The listing builds one solid part. Answer for the finished solid, in the listing's coordinates (mm). A direction names the side the tool comes from. Round coordinates to 2 decimals unless told otherwise and drop trailing zeros. Write each loop counter-clockwise with the first axis right and the second up, starting at its lowest first coordinate (ties: lowest second). Pieces come first, ordered by that corner, then holes. Notation, with made-up numbers: M 39.25,-8.75 L 86.25,-8.75 A28 ccw 86.25,23.25 Z; hole C 31,0 d9. An arc over 180 degrees is marked long. One line per item, written item: value. Start each with the question number.
(1) Section B-B (x = 124.5) is taken. Determine the outline of the cut face in (y, z).
(2) Given P1, Ø10, axis at y = 3.5, z = -20, coming from the -X side; P2, Ø5, axis at y = 17, z = -32, coming from the -X side; P3, Ø3, axis at x = 81, y = 16, coming from the -Z side, each flat-ended and moving along its own axis, determine where each tip first touches the part or whether it passes through.
(3) Section D-D (z = -42) is taken. Determine the outline of the cut face in (x, y) (3 decimals), plus the area to 3 significant figures.
(4) Section C-C (y = 15.25) is taken. Determine the outline of the cut face in (x, z).
(5) Consider probe 1 along Y at (x, z) = (46.5, -7); probe 2 along X at (y, z) = (15, -19); probe 3 along Z at (x, y) = (181.5, 18.25). Determine where each line is inside the solid, lowest interval first.
(6) Section A-A (z = -10) is taken. Determine the outline of the cut face in (x, y) (3 decimals).
(7) For faces 1 (the flat face through (32.766, 16, -35)), 2 (the flat face through (126, 16, -52.07)), 3 (the flat face through (128, 16, -18.288)), determine the directions among +Z, -Z, +X, -X, +Y, -Y from which every point of the face is accessible in a straight line to the end or side of a thin tool.
```python
from build123d import *

# Parameters (mm, degrees)
SKETCH1_W           = 254
SKETCH1_H           = 58.42
BOSS_EXTRUDE1_DEPTH = 19.05
CUT_EXTRUDE1_DEPTH  = 6.35
FILLET1_R           = 9.525


with BuildPart() as part:
    # Sketch1 → Boss-Extrude1 (new body)
    with BuildSketch(Plane(origin=(0, 0, 0), x_dir=(1, 0, 0), z_dir=(0, 1, 0))):
        with Locations((127, 29.21)):
            Rectangle(SKETCH1_W, SKETCH1_H)
    extrude(amount=BOSS_EXTRUDE1_DEPTH)

    # Sketch2 → Cut-Extrude1 (cut)
    with BuildSketch(Plane(origin=(0, 19.05, 0), x_dir=(1, 0, 0), z_dir=(0, 1, 0))):
        Polygon((221.234, 52.07), (221.234, 18.288), (127, 18.288), (127, 0), (254, 0), (254, 58.42), (127, 58.42), (127, 52.07), align=None)
        Polygon((127, 0), (127, 18.288), (32.766, 18.288), (32.766, 52.07), (127, 52.07), (127, 58.42), (0, 58.42), (0, 0), align=None)
    extrude(amount=-CUT_EXTRUDE1_DEPTH, mode=Mode.SUBTRACT)

    # Fillet1
    fillet1_edges = [part.edges().sort_by_distance(p)[0] for p in [
        (254, 0, -29.21),
        (0, 0, -29.21),
    ]]
    fillet(fillet1_edges, radius=FILLET1_R)


solid = part.part
```
Recorded:
1. outline: M 0,-58.42 L 12.7,-58.42 L 12.7,-52.07 L 19.05,-52.07 L 19.05,-18.29 L 12.7,-18.29 L 12.7,0 L 0,0 Z
2. P1: stops at x = 0.06
2. P2: stops at x = 32.77
2. P3: stops at z = -52.07
3. outline: M 0,9.525 A9.525 ccw 9.525,0 L 244.475,0 A9.525 ccw 254,9.525 L 254,12.7 L 221.234,12.7 L 221.234,19.05 L 32.766,19.05 L 32.766,12.7 L 0,12.7 Z
3. area: 4,380 mm2
4. outline: M 32.77,-52.07 L 221.23,-52.07 L 221.23,-18.29 L 32.77,-18.29 Z
5. probe 1: y = 0 to 12.7
5. probe 2: x = 32.77 to 221.23
5. probe 3: z = -52.07 to -18.29
6. outline: M 0,9.525 A9.525 ccw 9.525,0 L 244.475,0 A9.525 ccw 254,9.525 L 254,12.7 L 0,12.7 Z
7. face 1: +Z, -Z, -X, +Y
7. face 2: -Z, +X, -X, +Y
7. face 3: +Z, +X, -X, +Y
